```python
from build123d import *

# Parameters (mm, degrees)
EXTRUDE_305_DEPTH = 10
SKETCH_2_R        = 21
EXTRUDE_1_DEPTH   = 34
EXTRUDE_2_DEPTH   = 10


with BuildPart() as part:
    # Эскиз1 → Extrude 305 (new body)
    with BuildSketch(Plane(origin=(0, 0, 0), x_dir=(0, 0, -1), z_dir=(1, 0, 0))):
        Polygon((17.320508076, 0), (8.660254038, 15), (-8.660254038, 15), (-17.320508076, 0), (-8.660254038, -15), (8.660254038, -15), align=None)
    extrude(amount=EXTRUDE_305_DEPTH)

    # Эскиз2 → Бобышка-Вытянуть1 (add)
    with BuildSketch(Plane(origin=(10, 0, 0), x_dir=(0, 0, -1), z_dir=(1, 0, 0))):
        Circle(SKETCH_2_R)
    extrude(amount=EXTRUDE_1_DEPTH)

    # Эскиз3 → Бобышка-Вытянуть2 (add)
    with BuildSketch(Plane(origin=(44, 0, 0), x_dir=(0, 0, -1), z_dir=(1, 0, 0))):
        Polygon((17.320508076, 0), (8.660254038, 15), (-8.660254038, 15), (-17.320508076, 0), (-8.660254038, -15), (8.660254038, -15), align=None)
    extrude(amount=EXTRUDE_2_DEPTH)


solid = part.part
```
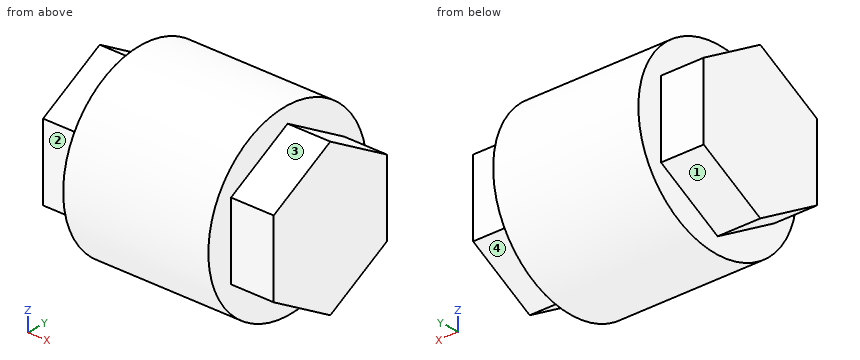
Part model, mm, in its own coordinate system. Face numbers are marked on the shaded views. A direction names the side the tool comes from. Round coordinates to 2 decimals unless told otherwise and drop trailing zeros. Loops run counter-clockwise (first coordinate to the right, second up) from the corner with the lowest first, then second, coordinate; pieces in that order, holes last. Notation, with made-up numbers: (87.25, -20.75) -> (141.25, -20.75) arc R20 ccw to (141.25, -7.75) -> close; hole circle Ø8 at (68, -21.5). An arc over 180 degrees is marked (long way). Use one line per item in the form item = value. Start each with the question number.
Item 1: Drop flat-ended pins along their axis: pin 1 Ø3 at (x, z) = (50, 4) entering from -Y; pin 2 Ø12 at (x, y) = (35, 15.5) entering from +Z; pin 3 Ø3 at (x, z) = (41, -13.5) entering from +Y. Give the stop position or say it passes through.
Item 2: Band-saw the part on D-D (z = -13.5). List the corners of the cut face in (x, y).
Item 3: Band-saw the part on B-B (x = 9). List the corners of the cut face in (y, z), plus the area to 3 significant figures.
Item 4: Drill centre lines: line 1 along X through (y, z) = (17, 1.5); line 2 along Y through (x, z) = (47, -3.5); line 3 along Y through (x, z) = (30, -12.5). Where is each one in solid material? Low to high.
Item 5: Tool access for the marked faces 1, 2, 3 and 4: list every direction of +Z, -Z, +X, -X, +Y, -Y with a clear straight run to the whole face (end or side of a thin tool).
Item 6: Band-saw the part on A-A (z = 0). List the corners of the cut face in (x, y), plus the area to 3 significant figures.
Item 7: Band-saw the part on C-C (y = 16). List the corners of the cut face in (x, z).
Data:
q1.pin_1 = -15
q1.pin_2 = 18.73
q1.pin_3 = 17.23
q2.outline = (0, -6.62) -> (10, -6.62) -> (10, -16.09) -> (44, -16.09) -> (44, -6.62) -> (54, -6.62) -> (54, 6.62) -> (44, 6.62) -> (44, 16.09) -> (10, 16.09) -> (10, 6.62) -> (0, 6.62) -> close
q3.outline = (-15, -8.66) -> (0, -17.32) -> (15, -8.66) -> (15, 8.66) -> (0, 17.32) -> (-15, 8.66) -> close
q3.area = 779 mm^2
q4.line_1 = 10 to 44
q4.line_2 = -15 to 15
q4.line_3 = -16.87 to 16.87
q5.face_1 = -Z, -X, +Y
q5.face_2 = +Z, -Z, -X, -Y
q5.face_3 = +Z, +X, -Y
q5.face_4 = -Z, +X, +Y
q6.outline = (0, -15) -> (10, -15) -> (10, -21) -> (44, -21) -> (44, -15) -> (54, -15) -> (54, 15) -> (44, 15) -> (44, 21) -> (10, 21) -> (10, 15) -> (0, 15) -> close
q6.area = 2,030 mm^2
q7.outline = (10, -13.6) -> (44, -13.6) -> (44, 13.6) -> (10, 13.6) -> close
